```python
from build123d import *

# Parameters (mm, degrees)
SKETCH1_R           = 30
SKETCH1_R_2         = 15
BOSS_EXTRUDE2_DEPTH = 40
BOSS_EXTRUDE8_DEPTH = 30
BOSS_EXTRUDE9_DEPTH = 20
RIB1_REACH          = 142.228
SKETCH10_WALL_W     = 344.295269622
SKETCH10_WALL_H     = 12


with BuildPart() as part:
    # Sketch1 → Boss-Extrude2 (new, symmetric)
    with BuildSketch(Plane(origin=(0, 0, 0), x_dir=(1, 0, 0), z_dir=(0, 1, 0))):
        with Locations(Location((0, 0, 0), (0, 0, 270))):
            Circle(SKETCH1_R)
        with Locations(Location((0, 0, 0), (0, 0, 270))):
            Circle(SKETCH1_R_2, mode=Mode.SUBTRACT)
    extrude(amount=BOSS_EXTRUDE2_DEPTH, both=True)

    # Sketch2 → Boss-Extrude8 (add, symmetric)
    with BuildSketch(Plane(origin=(0, 0, 0), x_dir=(1, 0, 0), z_dir=(0, 1, 0))):
        with BuildLine():
            Line((-30, 0), (-30, 48))
            Line((-30, 48), (-50, 48))
            Line((-50, 48), (-50, 68))
            Line((-50, 68), (-30, 68))
            Line((-30, 68), (-10, 68))
            Line((-10, 68), (-10, 28.284271247))
            ThreePointArc((-10, 28.284271247), (-24.494897428, 17.320508076), (-30, 0))
        make_face()
    extrude(amount=BOSS_EXTRUDE8_DEPTH, both=True)

    # Sketch7 → Boss-Extrude9 (add)
    with BuildSketch(Plane(origin=(0, 0, -68), x_dir=(-1, 0, 0), z_dir=(0, 0, -1))):
        with BuildLine():
            Line((50, 30), (50, -30))
            ThreePointArc((50, -30), (80, 0), (50, 30))
        make_face()
    extrude(amount=-BOSS_EXTRUDE9_DEPTH)

    # Sketch9 → Revolve2 (revolve)
    with BuildSketch(Plane(origin=(0, 0, 0), x_dir=(1, 0, 0), z_dir=(0, 1, 0)), mode=Mode.PRIVATE) as revolve2_sk:
        Polygon((-80, 68), (-70, 108), (-60, 108), (-60, 68), align=None)
    revolve(revolve2_sk.sketch.rotate(Axis((-50, 0, -68), (0, 0, -1)), 180), axis=Axis((-50, 0, -68), (0, 0, -1)))

    # Sketch10 wall → Rib1 (add, up to next)
    with BuildSketch(Plane(origin=(7.39950663, 0, -42.441103916), x_dir=(0.562740261082, 0, 0.826633775355), z_dir=(0.826633775355, 0, -0.562740261082)), mode=Mode.PRIVATE) as rib1_sk1:
        Rectangle(SKETCH10_WALL_W, SKETCH10_WALL_H)
    rib1_tool1 = extrude(rib1_sk1.sketch, amount=-RIB1_REACH, mode=Mode.PRIVATE) - part.part
    add(rib1_tool1.solids().sort_by_distance((7.39950663, 0, -42.441103916))[0])


solid = part.part
```
Source: CAD feature listing. Evaluate the final solid. Frame: model axes, mm. A direction names the side the tool comes from. Give positions to 0.01 mm unless a question says otherwise; leave off trailing zeros. Loops run counter-clockwise (first coordinate to the right, second up) from the corner with the lowest first, then second, coordinate; pieces in that order, holes last. Notation, with made-up numbers: (11.5, 51.5) -> (33.5, 51.5) arc R31 ccw to (33.5, 79.5) -> close; hole circle Ø10 at (53, 36.5). An arc over 180 degrees is marked (long way). Put each result on its own line as item: value. Start each with the question number.
1) Cut plane B-B (y = 0). Return loops of the section in (x, z), then the cut area to 3 significant figures.
2) Cut plane D-D (z = -84). Return loops of the section in (x, y).
3) Cut plane C-C (x = 9). Return loops of the section in (y, z), then the cut area to 3 significant figures.
4) Contact query for flat-ended pins moving along their axis: P1, Ø25, axis at x = -63, y = 5.5, coming from the +Z side; P2, Ø4, axis at y = -4, z = -76.5, coming from the +X side; P3, Ø6, axis at x = -52, y = 2, coming from the -Z side; P4, Ø24, axis at x = 0, z = 0, coming from the -Y side. Output: stop coordinate, or through.
5) Cut plane A-A (z = -4). Return loops of the section in (x, y), then the cut area to 3 significant figures.
6) Draft query along Z for faces 1 (the face through (-27.28, -7.15, -92.72)), 2 (the face through (-60, 0, -88)), 3 (the face through (0.66, -0.56, -14.985)). Return one class per face: released by +Z, released by -Z, zero draft, split by the parting line, or undercut.
7) Material intervals for probe 1 along X at (y, z) = (-6.5, 0); probe 2 along Y at (x, z) = (-49, -60); probe 3 along Z at (x, y) = (-12.5, -27), sorted ascending.
8) Reachability of faces 4 (the face through (-30, 0, -24)), 5 (the face through (-25, 30, -50)), 6 (the face through (-25, -30, -50)), 7 (the face through (-50, 0, -68)) from +Z, -Z, +X, -X, +Y, -Y: full face, straight path, thin tool, end or side. Return the list, or none.
Results are:
1. outline: (-80, -68) -> (-70, -108) -> (-60, -108) -> (-60, -68) -> (-40, -68) -> (-40, -108) -> (-30, -108) -> (-20, -68) -> (-10, -68) -> (24.8, -16.88) arc R30 ccw (long way) to (-30, 0) -> (-30, -48) -> (-80, -48) -> close; hole circle Ø30 at (0, 0)
1. area: 5,800 mm2
2. outline: circle Ø52 at (-50, 0); hole circle Ø20 at (-50, 0)
3. outline: (-40, -28.62) -> (-6, -28.62) -> (-6, -40.09) -> (6, -40.09) -> (6, -28.62) -> (40, -28.62) -> (40, -12) -> (-40, -12) -> close; (-40, 12) -> (40, 12) -> (40, 28.62) -> (-40, 28.62) -> close
3. area: 2,800 mm2
4. P1: stops at z = -48
4. P2: stops at x = -21.85
4. P3: stops at z = -68
4. P4: passes through
5. outline: (-30, -30) -> (-29.73, -30) -> (-29.73, -40) -> (-14.46, -40) -> (-14.46, 40) -> (-29.73, 40) -> (-29.73, 30) -> (-30, 30) -> close; (14.46, -40) -> (29.73, -40) -> (29.73, 40) -> (14.46, 40) -> close
5. area: 2,460 mm2
6. face 1: released by -Z
6. face 2: zero draft
6. face 3: undercut
7. probe 1: x = -30 to -15, 15 to 30
7. probe 2: y = -30 to 30
7. probe 3: z = -68 to -8.29, 8.29 to 27.27
8. face 4: +Z, -X, +Y, -Y
8. face 5: -Z, -X, +Y
8. face 6: -Z, -X, -Y
8. face 7: -Z
